Model file for the job. Use its own axes, mm. A direction names the side the tool comes from. Round coordinates to 2 decimals unless told otherwise and drop trailing zeros. Loops run counter-clockwise (first coordinate to the right, second up) from the corner with the lowest first, then second, coordinate; pieces in that order, holes last. Notation, with made-up numbers: M 35,12.5 L 76,12.5 A36 ccw 76,49.5 Z; hole C -38.5,51.25 d4. An arc over 180 degrees is marked long. Use a Markdown table: item, result. Add a question column.
Item 1: Saw through at C-C on z = -6.5. Write the cut outline in (x, y) (1 decimal), then the cut area to 3 significant figures.
Item 2: Pin check, flat tip, straight feed: P1, Ø8, axis at x = 47, z = -16.5, coming from the -Y side. Stop position of the tip, or through.
Item 3: Tool access for faces 1 (the flat face through (63.5, 27, -24)), 2 (the cylindrical face through (14.28, -3.68, -23.83)), 3 (the flat face through (14, -25, -3.175)): list every direction of +Z, -Z, +X, -X, +Y, -Y with a clear straight run to the whole face (end or side of a thin tool).
Item 4: Wall check: L1, parallel to Y at x = 75, z = -12.7 (1 decimal); L2, parallel to X at y = -22, z = -10.5 (3 decimals); L3, parallel to Z at x = 69, y = -6.5 (3 decimals). Give the ranges that are in metal, low to high. Write a range as from..to.
Item 5: Saw through at A-A on y = 27.94. Write the cut outline in (x, z) (3 decimals).
Item 6: Saw through at D-D on x = 38.1. Write the cut outline in (y, z) (3 decimals).
Item 7: Two-plate mould, pull along X, no slides. Class faces 4 (the flat face through (12, -7, -25.4)), 5 (the flat face through (0, -7, -13)), 6 (the flat face through (3.175, -47, -13)): +X half, -X half, draft (parallel to the pull), parting line (faces both ways), or undercut.
Item 8: Saw through at B-B on z = -12.7. Give the number of separate pieces and of enclosed holes in the cut face, then the cut area to 3 significant figures.
```python
from build123d import *

# Parameters (mm, degrees)
SKETCH1_W           = 76.2
SKETCH1_H           = 25.4
SKETCH1_W_2         = 69.85
SKETCH1_H_2         = 19.05
EXTRUDE_THIN1_DEPTH = 49.276
SKETCH2_R           = 2.4892
SKETCH2_R_2         = 24.97201
CUT_EXTRUDE1_DEPTH  = 52.578
CUT_EXTRUDE2_DEPTH  = 26.4
SKETCH6_R           = 3.175
CUT_EXTRUDE3_DEPTH  = 77.2
SKETCH7_R           = 3.175
CUT_EXTRUDE4_DEPTH  = 77.2


with BuildPart() as part:
    # Sketch1 → Extrude-Thin1 (new body, symmetric)
    with BuildSketch(Plane(origin=(0, 0, 0), x_dir=(1, 0, 0), z_dir=(0, 1, 0))):
        with Locations((38.1, 12.7)):
            Rectangle(SKETCH1_W, SKETCH1_H)
        with Locations((38.1, 12.7)):
            Rectangle(SKETCH1_W_2, SKETCH1_H_2, mode=Mode.SUBTRACT)
    extrude(amount=EXTRUDE_THIN1_DEPTH, both=True)

    # Sketch2 → Cut-Extrude1 (cut)
    with BuildSketch(Plane(origin=(0, 0, -25.4), x_dir=(-1, 0, 0), z_dir=(0, 0, -1))):
        with Locations((-5.2832, 21.6408)):
            Circle(SKETCH2_R)
        with Locations((-38.1, -11.176)):
            Circle(SKETCH2_R_2)
        with Locations((-70.9168, -43.9928)):
            Circle(SKETCH2_R)
    cut_extrude1 = extrude(amount=-CUT_EXTRUDE1_DEPTH, mode=Mode.SUBTRACT)

    # Sketch5 → Cut-Extrude2 (cut, through all)
    with BuildSketch(Plane(origin=(0, 0, -25.4), x_dir=(-1, 0, 0), z_dir=(0, 0, -1))):
        Polygon((0, 49.276), (-76.2, 49.276), (-76.2, 34.9885), (-63.5, 34.9885), (-12.7, 34.9885), (0, 34.9885), align=None)
        with BuildLine():
            Line((-12.7, 34.9885), (-63.5, 34.9885))
            Line((-63.5, 34.9885), (-63.5, 19.241588866))
            ThreePointArc((-63.5, 19.241588866), (-61.762611537, 16.410705953), (-58.451875232, 16.677992057))
            ThreePointArc((-58.451875232, 16.677992057), (-38.1, 23.32101), (-17.748124768, 16.677992057))
            ThreePointArc((-17.748124768, 16.677992057), (-14.437388463, 16.410705953), (-12.7, 19.241588866))
            Line((-12.7, 19.241588866), (-12.7, 34.9885))
        make_face()
    extrude(amount=-CUT_EXTRUDE2_DEPTH, mode=Mode.SUBTRACT)

    # Sketch6 → Cut-Extrude3 (cut, through all)
    with BuildSketch(Plane.ZY):
        with Locations((-12.7, 27.94)):
            Circle(SKETCH6_R)
    extrude(amount=-CUT_EXTRUDE3_DEPTH, mode=Mode.SUBTRACT)

    # Mirror1: Cut-Extrude1 across plane
    add(cut_extrude1.mirror(Plane.ZY.offset(-38.1)), mode=Mode.SUBTRACT)

    # Sketch7 → Cut-Extrude4 (cut, through all)
    with BuildSketch(Plane.ZY):
        with Locations((-12.7, -11.176)):
            Circle(SKETCH7_R)
    extrude(amount=-CUT_EXTRUDE4_DEPTH, mode=Mode.SUBTRACT)


solid = part.part
```
Entries:
| question | item | result |
|---|---|---|
| 1 | outline | M 0,-49.3 L 3.2,-49.3 L 3.2,-45.3 A2.5 cw 3.2,-42.7 L 3.2,20.3 A2.5 cw 3.2,23 L 3.2,35 L 0,35 Z; M 73,-49.3 L 76.2,-49.3 L 76.2,35 L 73,35 L 73,23 A2.5 cw 73,20.3 L 73,-42.7 A2.5 cw 73,-45.3 Z |
| 1 | area | 532 mm2 |
| 2 | P1 | through |
| 3 | face 1 | +Z, -Z, +Y |
| 3 | face 2 | +Z, -Z |
| 3 | face 3 | +Y, -Y |
| 4 | L1 | -49.3..-14.4, -8..24.8, 31.1..35 |
| 4 | L2 | 0..3.175, 73.025..76.2 |
| 4 | L3 | -25.4..-22.225, -3.175..0 |
| 5 | outline | M 0,-25.4 L 12.7,-25.4 L 12.7,-22.225 L 3.175,-22.225 L 3.175,-15.875 L 0,-15.875 Z; M 0,-9.525 L 3.175,-9.525 L 3.175,-3.175 L 12.7,-3.175 L 12.7,0 L 0,0 Z; M 63.5,-25.4 L 76.2,-25.4 L 76.2,-15.875 L 73.025,-15.875 L 73.025,-22.225 L 63.5,-22.225 Z; M 63.5,-3.175 L 73.025,-3.175 L 73.025,-9.525 L 76.2,-9.525 L 76.2,0 L 63.5,0 Z |
| 6 | outline | M -49.276,-25.4 L -36.148,-25.4 L -36.148,-22.225 L -49.276,-22.225 Z; M -49.276,-3.175 L -36.148,-3.175 L -36.148,0 L -49.276,0 Z; M 13.796,-25.4 L 23.321,-25.4 L 23.321,-22.225 L 13.796,-22.225 Z; M 13.796,-3.175 L 23.321,-3.175 L 23.321,0 L 13.796,0 Z |
| 7 | face 4 | draft |
| 7 | face 5 | -X half |
| 7 | face 6 | undercut |
| 8 | separate pieces | 6 |
| 8 | enclosed holes | 0 |
| 8 | area | 452 mm2 |
